```python
from build123d import *

# Parameters (mm, degrees)
BOSS_EXTRUDE1_DEPTH = 20.32
CUT_EXTRUDE1_START  = -17.78
CUT_EXTRUDE1_DEPTH  = 17.78
SKETCH3_6_R         = 0.762
CUT_EXTRUDE2_DEPTH  = 13.97
SKETCH3_7_R         = 0.762
CUT_EXTRUDE3_DEPTH  = 13.97
SKETCH3_8_R         = 0.762
CUT_EXTRUDE4_DEPTH  = 13.97
SKETCH3_9_R         = 0.762
CUT_EXTRUDE5_DEPTH  = 13.97


with BuildPart() as part:
    # Sketch1 → Boss-Extrude1 (new body)
    with BuildSketch(Plane.XY):
        with BuildLine():
            Line((-8.001, 16.383), (9.017, 16.383))
            ThreePointArc((9.017, 16.383), (11.98048452, 15.15548452), (13.208, 12.192))
            Line((13.208, 12.192), (13.208, -4.826))
            ThreePointArc((13.208, -4.826), (11.98048452, -7.78948452), (9.017, -9.017))
            Line((9.017, -9.017), (-8.001, -9.017))
            ThreePointArc((-8.001, -9.017), (-10.96448452, -7.78948452), (-12.192, -4.826))
            Line((-12.192, -4.826), (-12.192, 12.192))
            ThreePointArc((-12.192, 12.192), (-10.96448452, 15.15548452), (-8.001, 16.383))
        make_face()
        with BuildLine():
            Line((-5.461, -6.477), (5.461, -6.477))
            ThreePointArc((5.461, -6.477), (8.42448452, -5.24948452), (9.652, -2.286))
            Line((9.652, -2.286), (9.652, 2.286))
            ThreePointArc((9.652, 2.286), (8.42448452, 5.24948452), (5.461, 6.477))
            Line((5.461, 6.477), (-5.461, 6.477))
            ThreePointArc((-5.461, 6.477), (-8.42448452, 5.24948452), (-9.652, 2.286))
            Line((-9.652, 2.286), (-9.652, -2.286))
            ThreePointArc((-9.652, -2.286), (-8.42448452, -5.24948452), (-5.461, -6.477))
        make_face(mode=Mode.SUBTRACT)
    extrude(amount=BOSS_EXTRUDE1_DEPTH)

    # Sketch3 → Cut-Extrude1 (cut)
    with BuildSketch(Plane.XY.offset(20.32).offset(CUT_EXTRUDE1_START)):
        with BuildLine():
            Line((-9.652, 12.192), (-9.652, 2.286))
            ThreePointArc((-9.652, 2.286), (-8.42448452, 5.24948452), (-5.461, 6.477))
            Line((-5.461, 6.477), (5.461, 6.477))
            ThreePointArc((5.461, 6.477), (8.42448452, 5.24948452), (9.652, 2.286))
            Line((9.652, 2.286), (9.652, 3.683))
            Line((9.652, 3.683), (9.652, 12.192))
            ThreePointArc((9.652, 12.192), (8.484566704, 12.675566704), (8.001, 13.843))
            Line((8.001, 13.843), (-8.001, 13.843))
            ThreePointArc((-8.001, 13.843), (-8.484566704, 12.675566704), (-9.652, 12.192))
        make_face()
    extrude(amount=CUT_EXTRUDE1_DEPTH, mode=Mode.SUBTRACT)

    # Sketch3_6 → Cut-Extrude2 (cut)
    with BuildSketch(Plane.XY.offset(20.32)):
        with Locations(Location((-9.779, 13.97, 0), (0, 0, 180))):
            Circle(SKETCH3_6_R)
    extrude(amount=-CUT_EXTRUDE2_DEPTH, mode=Mode.SUBTRACT)

    # Sketch3_7 → Cut-Extrude3 (cut)
    with BuildSketch(Plane.XY.offset(20.32)):
        with Locations((10.795, 13.97)):
            Circle(SKETCH3_7_R)
    extrude(amount=-CUT_EXTRUDE3_DEPTH, mode=Mode.SUBTRACT)

    # Sketch3_8 → Cut-Extrude4 (cut)
    with BuildSketch(Plane.XY.offset(20.32)):
        with Locations(Location((10.795, -6.604, 0), (0, 0, 180))):
            Circle(SKETCH3_8_R)
    extrude(amount=-CUT_EXTRUDE4_DEPTH, mode=Mode.SUBTRACT)

    # Sketch3_9 → Cut-Extrude5 (cut)
    with BuildSketch(Plane.XY.offset(20.32)):
        with Locations((-9.779, -6.604)):
            Circle(SKETCH3_9_R)
    extrude(amount=-CUT_EXTRUDE5_DEPTH, mode=Mode.SUBTRACT)


solid = part.part
```
Input: part model. Units: mm. Frame: model coordinates. A direction names the side the tool comes from. Round coordinates to 2 decimals unless told otherwise and drop trailing zeros. Loops run counter-clockwise (first coordinate to the right, second up) from the corner with the lowest first, then second, coordinate; pieces in that order, holes last.
1) Section query D-D on y = 7. Return the cut outline in (x, z).
Ans:
outline: (-12.19, 0) - (13.21, 0) - (13.21, 20.32) - (9.65, 20.32) - (9.65, 2.54) - (-9.65, 2.54) - (-9.65, 20.32) - (-12.19, 20.32) - close
2) Set-up query: faces 1 (the cylindrical face through (10.696, 14.726, 13.433)), 2 (the flat face through (0, -6.477, 10)), 3 (the cylindrical face through (11.948, 15.188, 10.018)). Return all of +Z, -Z, +X, -X, +Y, -Y with unobstructed straight access to the full face (end or side cutting, diameter ignored); none if empty.
Ans:
face 1: +Z
face 2: +Z, -Z
face 3: +Z, -Z, +X, +Y
3) Section query C-C on z = 3. Return the cut outline in (x, y).
Ans:
outline: (-12.19, -4.83) arc R4.19 ccw to (-8, -9.02) - (9.02, -9.02) arc R4.19 ccw to (13.21, -4.83) - (13.21, 12.19) arc R4.19 ccw to (9.02, 16.38) - (-8, 16.38) arc R4.19 ccw to (-12.19, 12.19) - close; hole (-9.65, -2.29) arc R4.19 ccw to (-5.46, -6.48) - (5.46, -6.48) arc R4.19 ccw to (9.65, -2.29) - (9.65, 12.19) arc R1.65 cw to (8, 13.84) - (-8, 13.84) arc R1.65 cw to (-9.65, 12.19) - close
4) Pull-direction query (Y, two-part tool) for faces 4 (the flat face through (13.208, 4, 10)), 5 (the cylindrical face through (12.01, -7.76, 10.02)), 6 (the flat face through (0, 6.477, 1)); classes: released by +Y, released by -Y, zero draft, split by the parting line, or undercut.
Ans:
face 4: zero draft
face 5: released by -Y
face 6: undercut
5) Pin query (flat end, axial travel): pin 1 (1.2 mm diameter, centred on x = 11, y = -6.5, fed in from +Z); pin 2 (0.8 mm diameter, centred on x = 10.5, y = 14, fed in from +Z); pin 3 (6 mm diameter, centred on x = 2, y = 7.5, fed in from +Z). Return the tip coordinate at first contact, or that it passes through.
Ans:
pin 1: stops at z = 20.32
pin 2: stops at z = 6.35
pin 3: stops at z = 2.54
6) Material intervals for line 1 (X direction, y = 3.75, z = 15.5); line 2 (Y direction, x = 0.25, z = 5); line 3 (Y direction, x = 11.25, z = 7.75), sorted ascending.
Ans:
line 1: x = -12.19 to -9.65, 9.65 to 13.21
line 2: y = -9.02 to -6.48, 13.84 to 16.38
line 3: y = -8.37 to -7.22, -5.99 to 13.36, 14.58 to 15.74
7) Section query B-B on y = -2.75. Return the cut outline in (x, z).
Ans:
outline: (-12.19, 0) - (-9.63, 0) - (-9.63, 20.32) - (-12.19, 20.32) - close; (9.63, 0) - (13.21, 0) - (13.21, 20.32) - (9.63, 20.32) - close
8) Section query A-A on x = 2.25. Return the cut outline in (y, z).
Ans:
outline: (-9.02, 0) - (-6.48, 0) - (-6.48, 20.32) - (-9.02, 20.32) - close; (6.48, 0) - (16.38, 0) - (16.38, 20.32) - (13.84, 20.32) - (13.84, 2.54) - (6.48, 2.54) - close
